Can you work these out from the model? Positions are in its coordinate system, mm. A direction names the side the tool comes from. Round coordinates to 2 decimals unless told otherwise and drop trailing zeros. Loops run counter-clockwise (first coordinate to the right, second up) from the corner with the lowest first, then second, coordinate; pieces in that order, holes last. Notation, with made-up numbers: (-15, 76.25) -> (32, 76.25) arc R18 ccw to (32, 82.25) -> close; hole circle Ø8 at (66, 10.5). An arc over 180 degrees is marked (long way). Answer as a JSON object with one key per item and string values.
Autodesk Inventor part; units mm, degrees
ref_plane "YZ Plane" through (0, 0, 0) normal (1, 0, 0) x (0, 1, 0)
ref_plane "XZ Plane" through (0, 0, 0) normal (0, 1, 0) x (-1, 0, 0)
ref_plane "XY Plane" through (0, 0, 0) normal (0, 0, 1) x (1, 0, 0)
sketch "Sketch1" plane through (0, 0, 0) normal (0, 1, 0) x (-1, 0, 0)
  line L0 (64.2981, 132.08) -> (64.2981, -172.72)
  line L1 (64.2981, -172.72) -> (29.3731, -172.72)
  line L2 (29.3731, -172.72) -> (29.3731, -164.4885)
  line L3 (64.2981, 132.08) -> (28.7381, 132.08)
  line L4 (28.7381, 132.08) -> (28.7381, 141.4156)
  line L5 (13.4981, 141.4156) -> (13.4981, 132.08)
  line L6 (13.4981, 132.08) -> (-22.0619, 132.08)
  line L7 (-22.0619, 132.08) -> (-22.0619, -172.72)
  line L8 (-22.0619, -172.72) -> (12.8631, -172.72)
  line L9 (12.8631, -172.72) -> (12.8631, -164.4885)
  arc A0 (28.7381, 141.4156) -> (13.4981, 141.4156) centre (21.1181, 157.48) ccw
  arc A1 (29.3731, -164.4885) -> (12.8631, -164.4885) centre (21.1181, -147.32) ccw
  point P0 (0, 0)
  dimension "d0" = 86.36
  dimension "d1" = 19.05
  dimension "d2" = 17.78
  dimension "d3" = 25.4
  dimension "d4" = 25.4
  dimension "d5" = 304.8
  dimension "d6" = 304.8
  dimension "d7" = 0
  dimension "d8" = 34.925
  dimension "d9" = 51.435
  dimension "d10" = 43.18
  dimension "d13" = 43.18
  dimension "d16" = 15.24
  dimension "d17" = 7.62
extrude "Extrusion1" add sketch "Sketch1" along normal blind 25.4
sketch "Sketch2" plane through (0, 25.4, 0) normal (0, 1, 0) x (1, 0, 0)
  line L0 (-64.2981, -132.08) -> (-28.7381, -132.08)
  line L1 (-13.4981, -132.08) -> (22.0619, -132.08)
  line L2 (-29.3731, 172.72) -> (-64.2981, 172.72)
  line L3 (22.0619, 172.72) -> (-12.8631, 172.72)
  line L4 (-64.2981, 172.72) -> (-64.2981, -132.08)
  line L5 (22.0619, -132.08) -> (22.0619, 172.72)
  line L6 (-54.1381, -132.08) -> (-54.1381, 172.72)
  line L7 (-64.2981, 172.72) -> (-29.3731, 172.72)
  line L8 (-45.2481, 172.72) -> (-45.2481, -132.08)
  line L9 (-54.1381, -132.08) -> (-45.2481, -132.08)
  line L10 (-54.1381, 172.72) -> (-45.2481, 172.72)
  line L11 (3.0119, -132.08) -> (3.0119, 172.72)
  line L12 (11.9019, 172.72) -> (11.9019, -132.08)
  line L13 (3.0119, -132.08) -> (11.9019, -132.08)
  line L14 (3.0119, 172.72) -> (11.9019, 172.72)
  point P0 (0, 0)
  dimension "d21" = 10.16
  dimension "d22" = 19.05
  dimension "d23" = 67.31
  dimension "d24" = 76.2
extrude "Extrusion2" cut sketch "Sketch2" against normal blind 4.7625 contours L6 L2 L8 L0 | L11 L3 L12 L1
fillet "Fillet1" radius 4.826 4 edges at (-28.7381, 12.7, 141.4156) (-13.4981, 12.7, 141.4156) (-29.3731, 12.7, -164.4885) (-12.8631, 12.7, -164.4885)
properties part number "Straight Track"
Q1. I want a section at A-A, the plane z = -147.32. Write out the boundary of the cut face in (x, y).
Determined:
{"outline": "(-64.3, 0) -> (-40.17, 0) -> (-40.17, 25.4) -> (-45.25, 25.4) -> (-45.25, 20.64) -> (-54.14, 20.64) -> (-54.14, 25.4) -> (-64.3, 25.4) -> close; (-2.07, 0) -> (22.06, 0) -> (22.06, 25.4) -> (11.9, 25.4) -> (11.9, 20.64) -> (3.01, 20.64) -> (3.01, 25.4) -> (-2.07, 25.4) -> close"}
Q2. I want a section at D-D, the plane x = 9. Write out the boundary of the cut face in (y, z), then the cut area to 3 significant figures.
Determined:
{"outline": "(0, -172.72) -> (20.64, -172.72) -> (20.64, 132.08) -> (0, 132.08) -> close", "area": "6,290 mm²"}
Q3. We'd pull the mould along Z, two halves only. Please class faces 4 (the flat face through (-50, 20.638, -22)), 5 (the flat face through (5, 13, -172.72)), 6 (the flat face through (-47, 13, 132.08)): pulls with the +Z half, pulls with the -Z half, needs draft (parallel to the pull), parting line crosses it, or undercut.
Determined:
{"face 4": "needs draft", "face 5": "pulls with the -Z half", "face 6": "undercut"}
Q4. If I drill on L1, parallel to X at y = 22, z = 65; L2, parallel to X at y = 17, z = -147.32; L3, parallel to Z at x = -11.5, y = 23, over which ranges is the centre line in solid material (lowest first)? Write a range as [from, to].
Determined:
{"L1": "[-64.3, -54.14], [-45.25, 3.01], [11.9, 22.06]", "L2": "[-64.3, -40.17], [-2.07, 22.06]", "L3": "[-172.72, -163.93], [-130.88, 132.08], [142.52, 172.43]"}
Q5. I'm going to push flat-ended pins straight in: pin 1 (2 mm diameter, centred on y = 11, z = 134.5, fed in from -X); pin 2 (7.5 mm diameter, centred on x = -1.5, y = 12.5, fed in from +Z); pin 3 (4.5 mm diameter, centred on x = -49, z = -74, fed in from +Y). Where does each tip first touch, or does it pass through?
Determined:
{"pin 1": "x = -28.74", "pin 2": "z = 165.5", "pin 3": "y = 20.64"}
Q6. I want a section at C-C, the plane z = 88.5. Write out the boundary of the cut face in (x, y).
Determined:
{"outline": "(-64.3, 0) -> (22.06, 0) -> (22.06, 25.4) -> (11.9, 25.4) -> (11.9, 20.64) -> (3.01, 20.64) -> (3.01, 25.4) -> (-45.25, 25.4) -> (-45.25, 20.64) -> (-54.14, 20.64) -> (-54.14, 25.4) -> (-64.3, 25.4) -> close"}
Q7. I want a section at B-B, the plane y = 8.5. Write out the boundary of the cut face in (x, z), then the cut area to 3 significant figures.
Determined:
{"outline": "(-64.3, -172.72) -> (-29.37, -172.72) -> (-29.37, -167.29) arc R4.83 ccw to (-31.56, -163.26) arc R19.05 cw (long way) to (-10.68, -163.26) arc R4.83 ccw to (-12.86, -167.29) -> (-12.86, -172.72) -> (22.06, -172.72) -> (22.06, 132.08) -> (-13.5, 132.08) -> (-13.5, 138.61) arc R4.83 cw to (-11.33, 142.64) arc R17.78 ccw (long way) to (-30.91, 142.64) arc R4.83 cw to (-28.74, 138.61) -> (-28.74, 132.08) -> (-64.3, 132.08) -> close", "area": "26,200 mm²"}
Q8. On a 3-axis mill with a long thin cutter (end or side, diameter ignored), from which of +Z, -Z, +X, -X, +Y, -Y can I reach the whole of each face in a straight line? I mean faces 1 (the flat face through (-28.738, 13, 135)), 2 (the flat face through (-12.863, 13, -170)), 3 (the flat face through (-13.498, 13, 135)). Say none if no direction works.
Determined:
{"face 1": "-X, +Y, -Y", "face 2": "-Z, +Y, -Y", "face 3": "+X, +Y, -Y"}
